Could you check a few things on this model? Use its own coordinates, in mm. Face numbers are marked on the shaded views. A direction names the side the tool comes from. Give positions to 0.01 mm unless a question says otherwise; leave off trailing zeros. Loops run counter-clockwise (first coordinate to the right, second up) from the corner with the lowest first, then second, coordinate; pieces in that order, holes last. Notation, with made-up numbers: (38, 47) - (68, 47) arc R37 ccw to (68, 86) - close; hole circle Ø2 at (29.5, 15.25). An arc over 180 degrees is marked (long way). Answer in a Markdown table with one row per item. Add a question column.
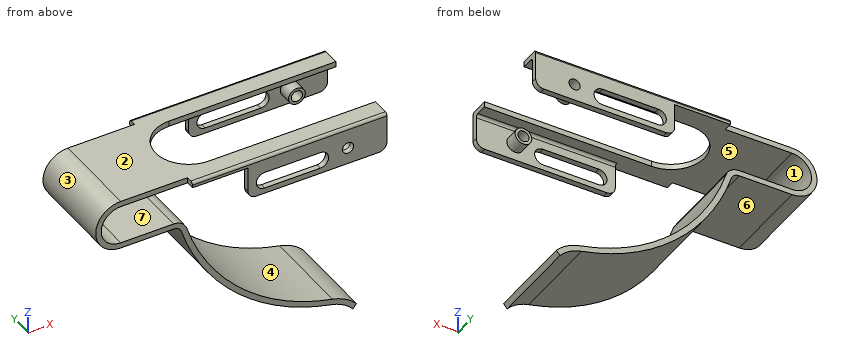
```python
from build123d import *

# Parameters (mm, degrees)
F1_DEPTH  = 16
F2_W      = 70
F2_H      = 3
F3_DEPTH  = 2
F4_W      = 50
F4_H      = 14
F5_DEPTH  = 2
F6_R      = 1
F9_DEPTH  = 2
F11_DEPTH = 38.001
F13_D     = 4
F14_R     = 3
F14_R_2   = 2
F15_DEPTH = 5
F16_R     = 3


# Not quite as in the source:
# - a pattern or mirror of a feature is missing from the dataset's text; its kind, count and spacing are read off the source's solid


with BuildPart() as f1:
    # F0 (on Front) → F1 (new body)
    with BuildSketch(Plane.XZ):
        with BuildLine():
            Line((94, 9), (0, 9))
            ThreePointArc((0, 9), (-9, 0), (0, -9))
            Line((0, -9), (19, -9))
            ThreePointArc((19, -9), (20.7747485708, -9.5812673752), (21.8617615127, -11.0998216597))
            ThreePointArc((21.8617615127, -11.0998216597), (42.1784205856, -42.831899352), (75.7404983282, -59.9572702431))
            ThreePointArc((75.7404983282, -59.9572702431), (79.997153255, -61.6128288571), (83.4944279816, -64.5503541724))
            Line((83.4944279816, -64.5503541724), (84.7953295958, -63))
            ThreePointArc((84.7953295958, -63), (80.8735692863, -59.8084227638), (76.1517077584, -58))
            ThreePointArc((76.1517077584, -58), (43.5219099532, -41.3503338559), (23.7696025212, -10.4997027661))
            ThreePointArc((23.7696025212, -10.4997027661), (21.9579142847, -7.9687789586), (19, -7))
            Line((19, -7), (0, -7))
            ThreePointArc((0, -7), (-7, 0), (0, 7))
            Line((0, 7), (94, 7))
            Line((94, 7), (94, 9))
        make_face()
    extrude(amount=F1_DEPTH)

    # F2 (on face) → F3 (join)
    with BuildSketch(Plane.XY.offset(9)):
        with Locations((59, -17.5)):
            Rectangle(F2_W, F2_H)
    extrude(amount=-F3_DEPTH)

    # F4 (on face) → F5 (join)
    with BuildSketch(Plane.XZ.offset(19)):
        with Locations((69, 2)):
            Rectangle(F4_W, F4_H)
    extrude(amount=-F5_DEPTH)

    # F6
    f6_edges = [f1.edges().sort_by_distance(p)[0] for p in [
        (59, -19, 9),
        (69, -17, 7),
    ]]
    fillet(f6_edges, radius=F6_R)

    # F7: F1 across plane


with BuildPart() as f1_1:
    add(f1.part)
    add(f1.part.mirror(Plane.XZ))

    # F8 (on face) → F9 (cut)
    with BuildSketch(Plane.XY.offset(9)):
        with BuildLine():
            Line((94, 12), (34, 12))
            ThreePointArc((34, 12), (22, 0), (34, -12))
            Line((34, -12), (94, -12))
            Line((94, -12), (94, 12))
        make_face()
    extrude(amount=-F9_DEPTH, mode=Mode.SUBTRACT)

    # F10 (on face) → F11 (cut, through all)
    with BuildSketch(Plane.XZ.offset(19)):
        with BuildLine():
            ThreePointArc((50, 3), (47, 0), (50, -3))
            Line((50, -3), (70, -3))
            ThreePointArc((70, -3), (73, 0), (70, 3))
            Line((70, 3), (50, 3))
        make_face()
    extrude(amount=-F11_DEPTH, mode=Mode.SUBTRACT)

    # F13 (through all)
    with Locations(Plane.XZ.offset(19)):
        with Locations((80, 1)):
            Hole(F13_D / 2)

    # F14 (on face) → F15 (join)
    with BuildSketch(Plane(origin=(0, -17, 0), x_dir=(-1, 0, 0), z_dir=(0, 1, 0))):
        with Locations((-80, 1)):
            Circle(F14_R)
        with Locations((-80, 1)):
            Circle(F14_R_2, mode=Mode.SUBTRACT)
    f15 = extrude(amount=F15_DEPTH)

    # F15_copies: F15 across plane
    add(f15.mirror(Plane.ZX))

    # F16
    f16_edges = [f1_1.edges().sort_by_distance(p)[0] for p in [
        (94, -18, -5),
        (94, 18, -5),
        (44, 18, -5),
        (44, -18, -5),
    ]]
    fillet(f16_edges, radius=F16_R)


solid = f1_1.part
```
(1) On a 3-axis mill with a long thin cutter (end or side, diameter ignored), from which of +Z, -Z, +X, -X, +Y, -Y can I reach the whole of each face in a straight line? I mean the marked faces 5, 6 and 7. Say none if no direction works.
(2) For pin 1 Ø2 at (x, y) = (56.5, 17.5) entering from -Z; pin 2 Ø12 at (x, z) = (76.5, -52) entering from +Y; pin 3 Ø2.5 at (y, z) = (-17, 3.5) entering from -X; pin 4 Ø3 at (x, z) = (80, 1) entering from +Y, each with a flat end and sliding along its axis, tell me the tip position at first contact or that it passes through.
(3) I want a section at C-C on z = 1. State how many separate pieces and enclosed holes the cut face has, then the cut area to 3 significant figures.
(4) I want a section at A-A on x = 42. Please give me the cut outline in (y, z).
(5) Please list where these lines run through material, in increasing order: line 1 (Y direction, x = 46.5, z = -3.5); line 2 (Z direction, x = 80, y = -14.95); line 3 (Z direction, x = 17, y = 12).
(6) I want a section at B-B on y = 0. Please give me the cut outline in (x, z), then the cut area to 3 significant figures.
(7) I want a section at D-D on y = -5.5. Please give me the cut outline in (x, z), then the cut area to 3 significant figures.
(8) We'd pull the mould along Z, two halves only. Please class the marked faces 1, 2, 3 and 4: pulls with the +Z half, pulls with the -Z half, needs draft (parallel to the pull), parting line crosses it, or undercut.
Reported:
| question | item | result |
|---|---|---|
| 1 | face 5 | none |
| 1 | face 6 | -Z, -X, +Y, -Y |
| 1 | face 7 | +X, +Y, -Y |
| 2 | pin 1 | z = -5 |
| 2 | pin 2 | y = 16 |
| 2 | pin 3 | x = -8.57 |
| 2 | pin 4 | through |
| 3 | separate pieces | 7 |
| 3 | enclosed holes | 0 |
| 3 | area | 166 mm² |
| 4 | outline | (-19, 7) - (-12, 7) - (-12, 9) - (-18, 9) arc R1 ccw to (-19, 8) - close; (-16, -42.67) - (16, -42.67) - (16, -39.93) - (-16, -39.93) - close; (12, 7) - (19, 7) - (19, 8) arc R1 ccw to (18, 9) - (12, 9) - close |
| 5 | line 1 | -19 to -17, 17 to 19 |
| 5 | line 2 | -61.61 to -59.34, -2 to -1, 3 to 4, 7 to 9 |
| 5 | line 3 | -9 to -7, 7 to 9 |
| 6 | outline | (0, -9) - (19, -9) arc R3 cw to (21.86, -11.1) arc R72 ccw to (75.74, -59.96) arc R14 cw to (83.49, -64.55) - (84.8, -63) arc R16 ccw to (76.15, -58) arc R70 cw to (23.77, -10.5) arc R5 ccw to (19, -7) - (0, -7) arc R7 cw to (0, 7) - (22, 7) - (22, 9) - (0, 9) arc R9 ccw to start |
| 6 | area | 312 mm² |
| 7 | outline | (0, -9) - (19, -9) arc R3 cw to (21.86, -11.1) arc R72 ccw to (75.74, -59.96) arc R14 cw to (83.49, -64.55) - (84.8, -63) arc R16 ccw to (76.15, -58) arc R70 cw to (23.77, -10.5) arc R5 ccw to (19, -7) - (0, -7) arc R7 cw to (0, 7) - (23.33, 7) - (23.33, 9) - (0, 9) arc R9 ccw to start |
| 7 | area | 315 mm² |
| 8 | face 1 | undercut |
| 8 | face 2 | pulls with the +Z half |
| 8 | face 3 | parting line crosses it |
| 8 | face 4 | undercut |
